Part print with two shaded views. Sizes in mm from the minimum x, y, z corner. A direction names the side the tool comes from. Round coordinates to 2 decimals unless told otherwise and drop trailing zeros. Loops run counter-clockwise (first coordinate to the right, second up) from the corner with the lowest first, then second, coordinate; pieces in that order, holes last. Notation, with made-up numbers: (31, 26) - (35, 26) arc R16 cw to (35, 33) - close; hole circle Ø8 at (-33.75, 29). An arc over 180 degrees is marked (long way). Use a Markdown table: item, result.
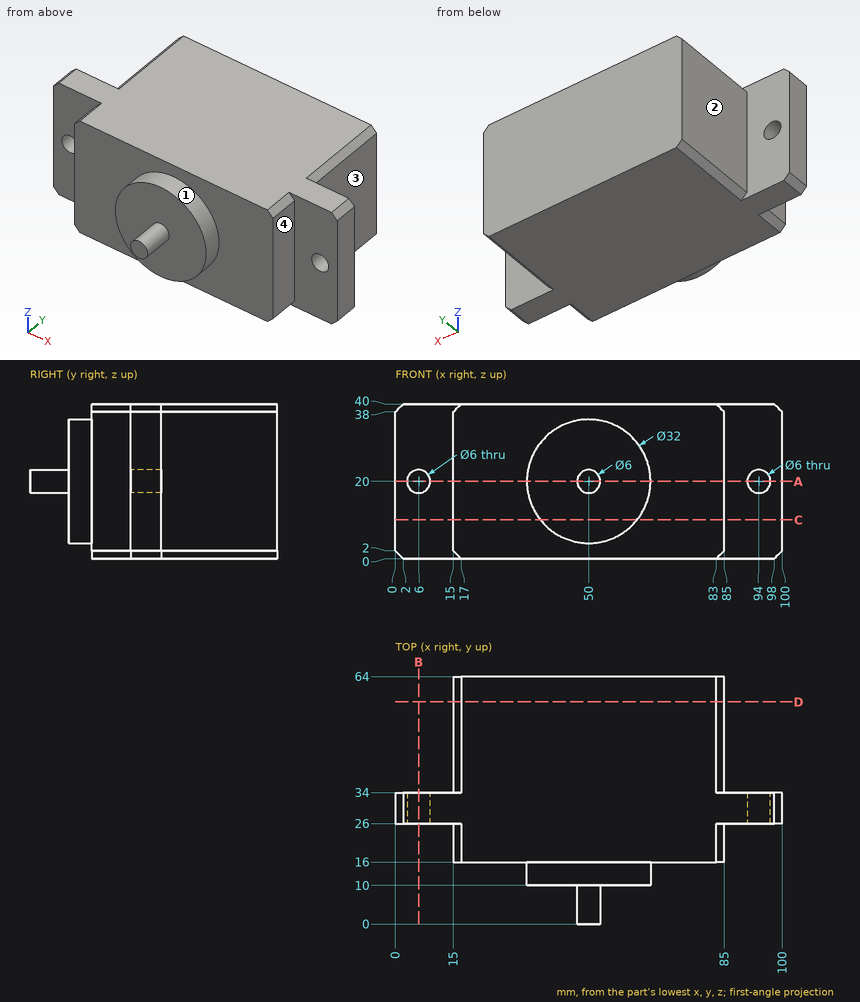
Q1. Cut at A-A, the plane z = 20. List the corners of the cut face in (x, y), plus the area to 3 significant figures.
Results found:
| item | result |
|---|---|
| outline | (0, 26) - (3, 26) - (3, 34) - (0, 34) - close; (9, 26) - (15, 26) - (15, 16) - (34, 16) - (34, 10) - (47, 10) - (47, 0) - (53, 0) - (53, 10) - (66, 10) - (66, 16) - (85, 16) - (85, 26) - (91, 26) - (91, 34) - (85, 34) - (85, 64) - (15, 64) - (15, 34) - (9, 34) - close; (97, 26) - (100, 26) - (100, 34) - (97, 34) - close |
| area | 3,760 mm2 |
Q2. Which spindle directions (+Z, -Z, +X, -X, +Y, -Y) get a long thin tool onto all of the face, cutting with end or side? Do the marked faces 1, 2, 3 and 4. Say none if no direction does.
Results found:
| item | result |
|---|---|
| face 1 | -Y |
| face 2 | +Z, -Z, -X, +Y |
| face 3 | +Z, -Z, +X, +Y |
| face 4 | +Z, -Z, +X, -Y |
Q3. Probe line 1 (Z direction, x = 94, y = 31); line 2 (Y direction, x = 83.5, z = 22); line 3 (Y direction, x = 8.5, z = 3.5). List the from-to ranges inside material, lowest first.
Results found:
| item | result |
|---|---|
| line 1 | z = 0 to 17, 23 to 40 |
| line 2 | y = 16 to 64 |
| line 3 | y = 26 to 34 |
Q4. Cut at B-B, the plane x = 6. List the corners of the cut face in (y, z), plus the area to 3 significant figures.
Results found:
| item | result |
|---|---|
| outline | (26, 0) - (34, 0) - (34, 17) - (26, 17) - close; (26, 23) - (34, 23) - (34, 40) - (26, 40) - close |
| area | 272 mm2 |
Q5. Cut at C-C, the plane z = 10. List the corners of the cut face in (x, y), plus the area to 3 significant figures.
Results found:
| item | result |
|---|---|
| outline | (0, 26) - (15, 26) - (15, 16) - (37.51, 16) - (37.51, 10) - (62.49, 10) - (62.49, 16) - (85, 16) - (85, 26) - (100, 26) - (100, 34) - (85, 34) - (85, 64) - (15, 64) - (15, 34) - (0, 34) - close |
| area | 3,750 mm2 |
Q6. Cut at D-D, the plane y = 57.5. List the corners of the cut face in (x, z).
Results found:
| item | result |
|---|---|
| outline | (15, 2) - (17, 0) - (83, 0) - (85, 2) - (85, 38) - (83, 40) - (17, 40) - (15, 38) - close |
Q7. Drop flat-ended pins along their axis: pin 1 (8 mm diameter, centred on x = 6, z = 20, fed in from +Y); pin 2 (1 mm diameter, centred on y = 14, z = 26, fed in from -X) (3 decimals); pin 3 (10 mm diameter, centred on x = 73, y = 8, fed in from +Z); pin 4 (9.5 mm diameter, centred on x = 94, z = 20, fed in from -Y). Give the stop position or say it passes through.
Results found:
| item | result |
|---|---|
| pin 1 | stops at y = 34 |
| pin 2 | stops at x = 34.975 |
| pin 3 | passes through |
| pin 4 | stops at y = 26 |
